For this review, take the finished solid that the model builds, in its own axes (mm). A direction names the side the tool comes from. Round coordinates to 2 decimals unless told otherwise and drop trailing zeros. Order: outer loops, then holes, each group sorted by start corner. A loop starts at its lowest first (then second) coordinate and runs counter-clockwise, first axis right, second up. Notation, with made-up numbers: M 79.25,-6.75 L 88.25,-6.75 A17 cw 88.25,26.25 Z; hole C 7,-22.5 d10. An arc over 180 degrees is marked long. Write item = value, one per line. Start each with the question number.
from build123d import *

# Parameters (mm, degrees)
SKETCH1_R           = 19
BOSS_EXTRUDE1_DEPTH = 35
SKETCH2_R           = 10
BOSS_EXTRUDE2_DEPTH = 5
SKETCH3_R           = 3
BOSS_EXTRUDE3_DEPTH = 13
CUT_EXTRUDE1_START  = -13
CUT_EXTRUDE1_DEPTH  = 13


with BuildPart() as part:
    # Sketch1 → Boss-Extrude1 (new body)
    with BuildSketch(Plane.XY):
        Circle(SKETCH1_R)
    extrude(amount=BOSS_EXTRUDE1_DEPTH)

    # Sketch2 → Boss-Extrude2 (add)
    with BuildSketch(Plane.XY.offset(35)):
        Circle(SKETCH2_R)
    extrude(amount=BOSS_EXTRUDE2_DEPTH)

    # Sketch3 → Boss-Extrude3 (add)
    with BuildSketch(Plane.XY.offset(40)):
        with Locations(Location((0, 0, 0), (0, 0, 180))):
            Circle(SKETCH3_R)
    extrude(amount=BOSS_EXTRUDE3_DEPTH)

    # Sketch4 → Cut-Extrude1 (cut)
    with BuildSketch(Plane.XY.offset(53).offset(CUT_EXTRUDE1_START)):
        with BuildLine():
            Line((-1.967057229, -2.265101733), (1.321836789, -2.693092554))
            ThreePointArc((1.321836789, -2.693092554), (-0.387132264, -2.974916572), (-1.967057229, -2.265101733))
        make_face()
    extrude(amount=CUT_EXTRUDE1_DEPTH, mode=Mode.SUBTRACT)


solid = part.part
(1) Insertion check: pin 1 (2 mm diameter, centred on y = -9, z = 25.5, fed in from -X); pin 2 (3 mm diameter, centred on x = -3.5, y = -10.5, fed in from +Z); pin 3 (1 mm diameter, centred on y = -9.5, z = 38.5, fed in from -X); pin 4 (6 mm diameter, centred on x = 1, y = 4.5, fed in from +Z). Each pin has a flat end and moves straight along its axis. Give the tip position at first contact, or say it passes through.
(2) For faces 1 (the flat face through (0, 0, 53)), 2 (the flat face through (2.1, 2.4, 40)), 3 (the flat face through (-0.346, -2.476, 46.409)), list the 3-axis set-ups (+Z, -Z, +X, -X, +Y, -Y) from which the entire face can be reached by the end or side of a thin tool; tool diameter is ignored.
(3) We need section B-B, the plane x = -8.5. Write out the cut boundary in (y, z).
(4) We need section C-C, the plane z = 43.5. Write out the cut boundary in (x, y).
(5) We need section D-D, the plane y = -5. Write out the cut boundary in (x, z).
(6) For line 1 along Z through (x, y) = (1, -14.5); line 2 along Z through (x, y) = (-3, -1); line 3 along Y through (x, z) = (-4, 24.5), list the stretches that pass through material, from the lowest coordinate up.
(7) We need section A-A, the plane y = 0. Write out the cut boundary in (x, z).
Values:
q1.pin_1 = -17.23
q1.pin_2 = 40
q1.pin_3 = -4.36
q1.pin_4 = 53
q2.face_1 = +Z, +X, -X, +Y, -Y
q2.face_2 = +Z
q2.face_3 = +Z, -X, -Y
q3.outline = M -16.99,0 L 16.99,0 L 16.99,35 L 5.27,35 L 5.27,40 L -5.27,40 L -5.27,35 L -16.99,35 Z
q4.outline = M -1.97,-2.27 L 1.32,-2.69 A3 ccw long Z
q5.outline = M -18.33,0 L 18.33,0 L 18.33,35 L 8.66,35 L 8.66,40 L -8.66,40 L -8.66,35 L -18.33,35 Z
q6.line_1 = 0 to 35
q6.line_2 = 0 to 40
q6.line_3 = -18.57 to 18.57
q7.outline = M -19,0 L 19,0 L 19,35 L 10,35 L 10,40 L 3,40 L 3,53 L -3,53 L -3,40 L -10,40 L -10,35 L -19,35 Z
